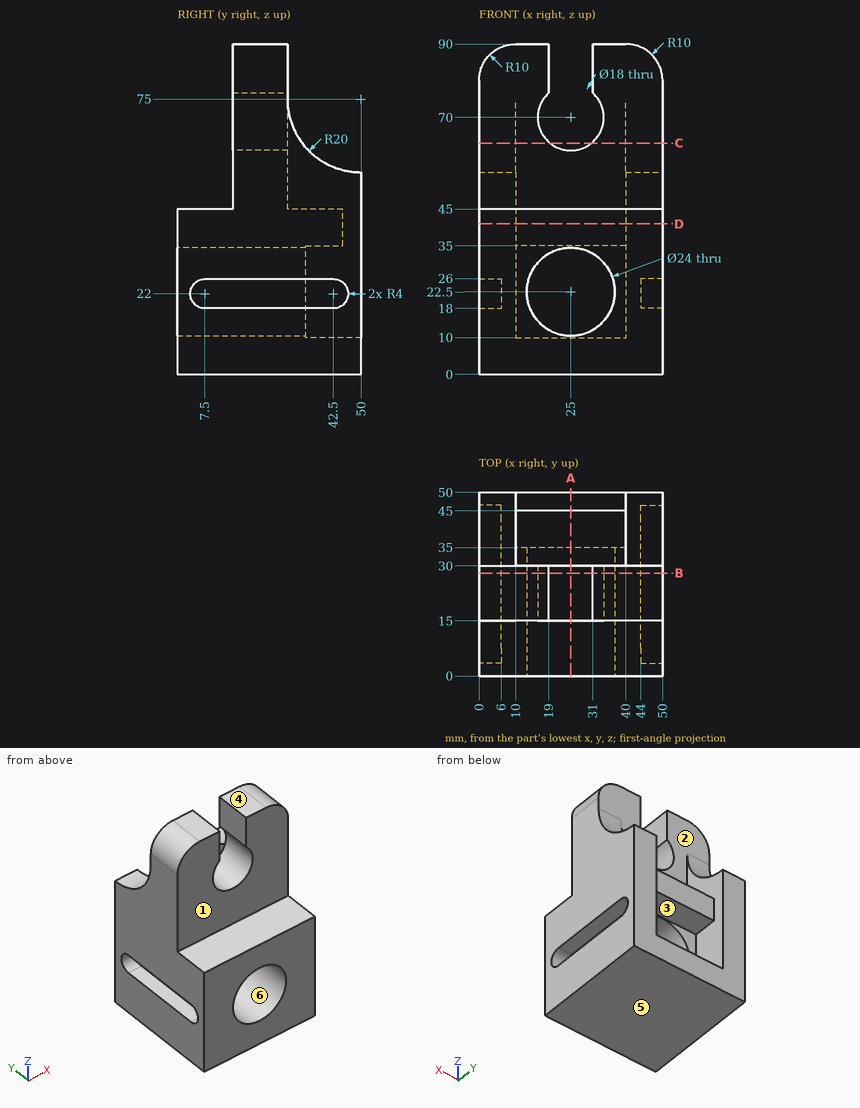
Input: dimensioned drawing with shaded views. Units: mm. Origin: part minimum x, y, z. A direction names the side the tool comes from. Round coordinates to 2 decimals unless told otherwise and drop trailing zeros. Order: outer loops, then holes, each group sorted by start corner. A loop starts at its lowest first (then second) coordinate and runs counter-clockwise, first axis right, second up.
1. Material intervals for line 1 (X direction, y = 26, z = 22); line 2 (X direction, y = 41, z = 20); line 3 (Y direction, x = 6.5, z = 77), sorted ascending.
The answers:
line 1: x = 6 to 13.01, 36.99 to 44
line 2: x = 6 to 10, 40 to 44
line 3: y = 15 to 30
2. Cut plane B-B, the plane y = 28. Output: boundary loops of the cut face in (x, z), then the cut area to 3 significant figures.
The answers:
outline: (0, 0) - (50, 0) - (50, 18) - (44, 18) - (44, 26) - (50, 26) - (50, 80) arc R10 ccw to (40, 90) - (31, 90) - (31, 76.71) arc R9 cw (long way) to (19, 76.71) - (19, 90) - (10, 90) arc R10 ccw to (0, 80) - (0, 26) - (6, 26) - (6, 18) - (0, 18) - close; hole circle Ø24 at (25, 22.5)
area: 3,510 mm2
3. Set-up query: the marked faces 1, 2 and 3. Return all of +Z, -Z, +X, -X, +Y, -Y with unobstructed straight access to the full face (end or side cutting, diameter ignored); none if empty.
The answers:
face 1: +Z, +X, -X, -Y
face 2: +Z, +Y
face 3: +Y
4. Cut plane D-D, the plane z = 41. Output: boundary loops of the cut face in (x, y).
The answers:
outline: (0, 0) - (50, 0) - (50, 50) - (40, 50) - (40, 45) - (10, 45) - (10, 50) - (0, 50) - close
5. Cut plane C-C, the plane z = 63. Output: boundary loops of the cut face in (x, y).
The answers:
outline: (0, 15) - (19.34, 15) - (19.34, 30) - (10, 30) - (10, 34) - (0, 34) - close; (30.66, 15) - (50, 15) - (50, 34) - (40, 34) - (40, 30) - (30.66, 30) - close
6. Mould query, pull axis Z, two halves, no side actions, for the marked faces 4, 5 and 6. Classes: released by +Z, released by -Z, zero draft, split by the parting line, or undercut.
The answers:
face 4: released by +Z
face 5: released by -Z
face 6: undercut
7. Cut plane A-A, the plane x = 25. Output: boundary loops of the cut face in (y, z).
The answers:
outline: (0, 0) - (50, 0) - (50, 10) - (35, 10) - (35, 10.5) - (0, 10.5) - close; (0, 34.5) - (35, 34.5) - (35, 35) - (45, 35) - (45, 45) - (30, 45) - (30, 61) - (15, 61) - (15, 45) - (0, 45) - close
8. Pin query (flat end, axial travel): P1, Ø1.5, axis at x = 8.5, z = 51, coming from the -Y side; P2, Ø1.5, axis at x = 15.5, z = 74, coming from the +Y side; P3, Ø6.5, axis at y = 23.5, z = 84.5, coming from the -X side. Return the tip coordinate at first contact, or that it passes through.
The answers:
P1: stops at y = 15
P2: stops at y = 30
P3: stops at x = 0.08
